```python
from build123d import *

# Parameters (mm, degrees)
F3_W     = 19.09311
F3_H     = 4.934694
F3_H_2   = 4.746388
F4_DEPTH = 4


with BuildPart() as f2:
    # F0 (on Right) → F2 (revolve)
    with BuildSketch(Plane.YZ):
        Polygon((-89.465849, 8), (-89.465849, 0), (-29.465849, 0), (-29.465849, 2), (-35.465849, 2), (-35.465849, 3), (-85.465849, 3), (-85.465849, 8), align=None)
    revolve(axis=Axis((0, -60.270485, 0), (0, 1, 0)))

    # F3 (on face) → F4 (cut, through all)
    with BuildSketch(Plane.XZ.offset(89.465849)):
        with Locations((0.222466, 7.467347)):
            Rectangle(F3_W, F3_H)
        with Locations((0.222466, -7.373194)):
            Rectangle(F3_W, F3_H_2)
    extrude(amount=-F4_DEPTH, mode=Mode.SUBTRACT)


solid = f2.part
```
Model file for the job. Use its own axes, mm. A direction names the side the tool comes from. Coordinates: 2 decimals unless noted, no trailing zeros. Order: outer loops, then holes, each group sorted by start corner. A loop starts at its lowest first (then second) coordinate and runs counter-clockwise, first axis right, second up. Notation, with made-up numbers: (14, 16.25) -> (25, 16.25) arc R24 ccw to (25, 37.25) -> close; hole circle Ø1 at (54.5, 62). An arc over 180 degrees is marked (long way). Answer as a JSON object with one key per item and string values. Group by question number.
1) Cut at A-A, the plane x = 0. Write the cut outline in (y, z).
2) Which spindle directions (+Z, -Z, +X, -X, +Y, -Y) get a long thin tool onto all of the face, cutting with end or side? Do faces 1 (the face through (0, -61, -3)), 2 (the face through (0, -87, -5)). Say none if no direction does.
3) Drill centre lines: L1, parallel to Y at x = 4.25, z = -2; L2, parallel to Z at x = -0.25, y = -65.5; L3, parallel to X at y = -85, z = 0. Where is each one in solid material? Low to high.
4) Flat gauge pins, fed straight in: pin 1 (1.5 mm diameter, centred on x = 4.5, y = -74, fed in from +Z); pin 2 (2 mm diameter, centred on y = -74.5, z = 2, fed in from -X); pin 3 (2 mm diameter, centred on x = -2.5, z = -2, fed in from +Y). Where does each tip first touch, or does it go through?
5) Cut at B-B, the plane z = 0. Write the cut outline in (x, y), then the cut area to 3 significant figures.
6) Cut at D-D, the plane z = -4. Write the cut outline in (x, y), then the cut area to 3 significant figures.
7) Cut at C-C, the plane y = -67. Write the cut outline in (x, z).
Check values:
{
 "1": {"outline": "(-89.47, -5) -> (-85.47, -5) -> (-85.47, -3) -> (-35.47, -3) -> (-35.47, -2) -> (-29.47, -2) -> (-29.47, 2) -> (-35.47, 2) -> (-35.47, 3) -> (-85.47, 3) -> (-85.47, 5) -> (-89.47, 5) -> close"},
 "2": {"face 1": "+Y", "face 2": "-Z, +X, -X, +Y, -Y"},
 "3": {"L1": "y = -89.47 to -85.47", "L2": "z = -2.99 to 2.99", "L3": "x = -3 to 3"},
 "4": {"pin 1": "passes through", "pin 2": "stops at x = -2.83", "pin 3": "stops at y = -35.47"},
 "5": {"outline": "(-8, -89.47) -> (8, -89.47) -> (8, -85.47) -> (3, -85.47) -> (3, -35.47) -> (2, -35.47) -> (2, -29.47) -> (-2, -29.47) -> (-2, -35.47) -> (-3, -35.47) -> (-3, -85.47) -> (-8, -85.47) -> close", "area": "388 mm²"},
 "6": {"outline": "(-6.93, -89.47) -> (6.93, -89.47) -> (6.93, -85.47) -> (-6.93, -85.47) -> close", "area": "55.4 mm²"},
 "7": {"outline": "circle Ø6 at (0, 0)"}
}
